```python
from build123d import *

# Parameters (mm, degrees)
F0_R     = 32.5
F1_DEPTH = 10
F2_R     = 8
F3_DEPTH = 25
F4_R     = 3.25
F5_DEPTH = 25
F6_T     = -2.5
F8_DEPTH = 25


with BuildPart() as f1:
    # F0 (on Top) → F1 (new body)
    with BuildSketch(Plane.XY):
        Circle(F0_R)
    extrude(amount=F1_DEPTH)

    # F2 (on Top) → F3 (cut)
    with BuildSketch(Plane.XY):
        Circle(F2_R)
    extrude(amount=F3_DEPTH, mode=Mode.SUBTRACT)

    # F4 (on face) → F5 (cut)
    with BuildSketch(Plane.XY.offset(10)):
        with Locations((-14.1421356237, 14.1421356237)):
            Circle(F4_R)
        with Locations((-14.1421356237, -14.1421356237)):
            Circle(F4_R)
        with Locations((14.1421356237, 14.1421356237)):
            Circle(F4_R)
        with Locations((14.1421356237, -14.1421356237)):
            Circle(F4_R)
    extrude(amount=-F5_DEPTH, mode=Mode.SUBTRACT)

    # F6
    f6_openings = [f1.faces().sort_by_distance(p)[0] for p in [
        (-31.580761, 0, 10),
    ]]
    offset(amount=F6_T, openings=f6_openings)

    # F7 (on face) → F8 (cut)
    with BuildSketch(Plane.XY.offset(2.5)):
        with BuildLine():
            ThreePointArc((19.8921356237, 14.1421356237), (19.0783691058, 11.1932207368), (16.8674055331, 9.0789939191))
            Line((16.8674055331, 9.0789939191), (26.4163915025, 14.218799527))
            ThreePointArc((26.4163915025, 14.218799527), (21.2132034356, 21.2132034356), (14.218799527, 26.4163915025))
            Line((14.218799527, 26.4163915025), (9.0789939191, 16.8674055331))
            ThreePointArc((9.0789939191, 16.8674055331), (15.5473820787, 19.7177775061), (19.8921356237, 14.1421356237))
        make_face()
        with BuildLine():
            Line((-9.0789939191, 16.8674055331), (-14.218799527, 26.4163915025))
            ThreePointArc((-14.218799527, 26.4163915025), (-21.2132034356, 21.2132034356), (-26.4163915025, 14.218799527))
            Line((-26.4163915025, 14.218799527), (-16.8674055331, 9.0789939191))
            ThreePointArc((-16.8674055331, 9.0789939191), (-18.2079996156, 18.2079996156), (-9.0789939191, 16.8674055331))
        make_face()
        with BuildLine():
            ThreePointArc((14.218799527, -26.4163915025), (21.2132034356, -21.2132034356), (26.4163915025, -14.218799527))
            Line((26.4163915025, -14.218799527), (16.8674055331, -9.0789939191))
            ThreePointArc((16.8674055331, -9.0789939191), (19.0783691058, -11.1932207368), (19.8921356237, -14.1421356237))
            ThreePointArc((19.8921356237, -14.1421356237), (15.5473820787, -19.7177775061), (9.0789939191, -16.8674055331))
            Line((9.0789939191, -16.8674055331), (14.218799527, -26.4163915025))
        make_face()
        with BuildLine():
            ThreePointArc((-26.4163915025, -14.218799527), (-21.2132034356, -21.2132034356), (-14.218799527, -26.4163915025))
            Line((-14.218799527, -26.4163915025), (-9.0789939191, -16.8674055331))
            ThreePointArc((-9.0789939191, -16.8674055331), (-18.2079996156, -18.2079996156), (-16.8674055331, -9.0789939191))
            Line((-16.8674055331, -9.0789939191), (-26.4163915025, -14.218799527))
        make_face()
    extrude(amount=-F8_DEPTH, mode=Mode.SUBTRACT)


solid = f1.part
```
Here's how the part is built. I have some questions about the finished solid (model axes, mm). A direction names the side the tool comes from. Coordinates: 2 decimals unless noted, no trailing zeros. Order: outer loops, then holes, each group sorted by start corner. A loop starts at its lowest first (then second) coordinate and runs counter-clockwise, first axis right, second up. Notation, with made-up numbers: (18.5, -16) -> (35.5, -16) arc R20 cw to (35.5, 11) -> close; hole circle Ø2 at (73.25, 70). An arc over 180 degrees is marked (long way). Return JSON: item names as keys, results as strings.
1) If we section it at A-A on z = 6.5: State how many separate pieces and enclosed holes the cut face has, plus the area to 3 significant figures.
Conclusion:
{"separate pieces": "6", "enclosed holes": "6", "area": "919 mm²"}
2) On a 3-axis mill with a long thin cutter (end or side, diameter ignored), from which of +Z, -Z, +X, -X, +Y, -Y can I reach the whole of each face in a straight line? I mean faces 1 (the flat face through (-12, -17, 10)), 2 (the flat face through (0, -13, 2.5)). Say none if no direction works.
Conclusion:
{"face 1": "+Z, +X, -X, +Y, -Y", "face 2": "+Z"}
3) If we section it at B-B on y = 0: List the corners of the cut face in (x, z) for me, plus the area to 4 significant figures.
Conclusion:
{"outline": "(-32.5, 0) -> (-8, 0) -> (-8, 10) -> (-10.5, 10) -> (-10.5, 2.5) -> (-30, 2.5) -> (-30, 10) -> (-32.5, 10) -> close; (8, 0) -> (32.5, 0) -> (32.5, 10) -> (30, 10) -> (30, 2.5) -> (10.5, 2.5) -> (10.5, 10) -> (8, 10) -> close", "area": "197.5 mm²"}
4) Thinking about a two-plate mould opening in X: for faces 3 (the cylindrical face through (31, 9.76, 4.93)), 4 (the cylindrical face through (10.895, 14.285, 5.07)), 5 (the flat face through (17, 12, 10)), which applies, +X half, -X half, draft (parallel to the pull), parting line (faces both ways), or undercut?
Conclusion:
{"face 3": "parting line", "face 4": "undercut", "face 5": "draft"}
5) If we section it at D-D on y = 13: List the corners of the cut face in (x, z) for me.
Conclusion:
{"outline": "(-29.79, 0) -> (-24.15, 0) -> (-24.15, 2.5) -> (-27.04, 2.5) -> (-27.04, 10) -> (-29.79, 10) -> close; (-19.78, 0) -> (-17.18, 0) -> (-17.18, 10) -> (-19.78, 10) -> close; (-11.1, 0) -> (11.1, 0) -> (11.1, 10) -> (8.51, 10) -> (8.51, 2.5) -> (-8.51, 2.5) -> (-8.51, 10) -> (-11.1, 10) -> close; (17.18, 0) -> (19.78, 0) -> (19.78, 10) -> (17.18, 10) -> close; (24.15, 0) -> (29.79, 0) -> (29.79, 10) -> (27.04, 10) -> (27.04, 2.5) -> (24.15, 2.5) -> close"}
6) I'm going to push flat-ended pins straight in: P1, Ø1, axis at x = -2, z = 4, coming from the -Y side; P2, Ø6, axis at x = 23.5, z = 3.5, coming from the -Y side; P3, Ø6, axis at x = -6.5, z = 5, coming from the +Y side. Where does each tip first touch, or does it pass through?
Conclusion:
{"P1": "stops at y = -32.47", "P2": "stops at y = -25.22", "P3": "stops at y = 32.31"}
7) If I drill on probe 1 along Y at (x, z) = (0, 6.75); probe 2 along Y at (x, z) = (6, 6); probe 3 along Y at (x, z) = (-23, 1.25), over which ranges is the centre line in solid material (lowest first)?
Conclusion:
{"probe 1": "y = -32.5 to -30, -10.5 to -8, 8 to 10.5, 30 to 32.5", "probe 2": "y = -31.94 to -29.39, -8.62 to -5.29, 5.29 to 8.62, 29.39 to 31.94", "probe 3": "y = -22.96 to -19.26, -12.38 to 12.38, 19.26 to 22.96"}
